from build123d import *

# Parameters (mm, degrees)
SKETCH1_R           = 50
BOSS_EXTRUDE2_DEPTH = 42
SKETCH2_R           = 4
CUT_EXTRUDE1_DEPTH  = 10
SKETCH3_W           = 20
SKETCH3_H           = 10
CUT_EXTRUDE3_DEPTH  = 5


with BuildPart() as part:
    # Sketch1 → Boss-Extrude2 (new body)
    with BuildSketch(Plane.XY):
        Circle(SKETCH1_R)
    extrude(amount=BOSS_EXTRUDE2_DEPTH)

    # Sketch2 → Cut-Extrude1 (cut)
    with BuildSketch(Plane(origin=(0, 0, 0), x_dir=(-1, 0, 0), z_dir=(0, 0, -1))):
        Circle(SKETCH2_R)
    extrude(amount=-CUT_EXTRUDE1_DEPTH, mode=Mode.SUBTRACT)

    # Sketch3 → Cut-Extrude3 (cut)
    with BuildSketch(Plane.XY.offset(42)):
        Rectangle(SKETCH3_W, SKETCH3_H)
    extrude(amount=-CUT_EXTRUDE3_DEPTH, mode=Mode.SUBTRACT)


solid = part.part
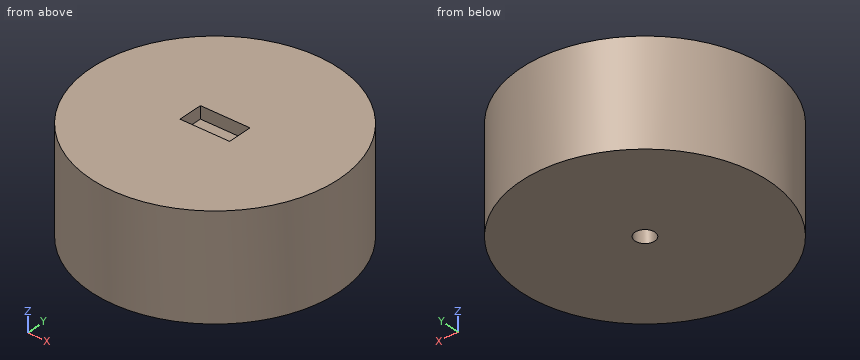
Read the model definition and answer for the solid it produces. Units are mm, in the model's axes. Round coordinates to 2 decimals unless told otherwise and drop trailing zeros. Order: outer loops, then holes, each group sorted by start corner. A loop starts at its lowest first (then second) coordinate and runs counter-clockwise, first axis right, second up.
1) The part is cut by section A-A on x = 0. Write down the section's boundary in (y, z).
2) The part is cut by section D-D on z = 35.5. Write down the section's boundary in (x, y).
3) Flat-ended cylindrical pins translate along their axes: pin 1 (2.5 mm diameter, centred on x = 3, z = 40, fed in from -Y); pin 2 (4 mm diameter, centred on x = -27, z = 9, fed in from -Y); pin 3 (12 mm diameter, centred on y = -39, z = 37, fed in from -X). Find the tip coordinate at first contact, or state that the pin passes through.
4) The part is cut by section C-C on z = 3. Write down the section's boundary in (x, y), plus the area to 3 significant figures.
5) The part is cut by section B-B on y = 0. Write down the section's boundary in (x, z), plus the area to 3 significant figures.
6) Straight lines are drawn through the part: L1, parallel to Y at x = 0, z = 6.25; L2, parallel to Z at x = 1, y = 2; L3, parallel to Y at x = 11.5, z = 28. For each, find the intervals that lie inside material, in ascending order.
Resolved:
1. outline: (-50, 0) - (-4, 0) - (-4, 10) - (4, 10) - (4, 0) - (50, 0) - (50, 42) - (5, 42) - (5, 37) - (-5, 37) - (-5, 42) - (-50, 42) - close
2. outline: circle Ø100 at (0, 0)
3. pin 1: stops at y = -49.97
3. pin 2: stops at y = -43.3
3. pin 3: stops at x = -37.56
4. outline: circle Ø100 at (0, 0); hole circle Ø8 at (0, 0)
4. area: 7,800 mm2
5. outline: (-50, 0) - (-4, 0) - (-4, 10) - (4, 10) - (4, 0) - (50, 0) - (50, 42) - (10, 42) - (10, 37) - (-10, 37) - (-10, 42) - (-50, 42) - close
5. area: 4,020 mm2
6. L1: y = -50 to -4, 4 to 50
6. L2: z = 10 to 37
6. L3: y = -48.66 to 48.66
